Geometry check sheet. Reference: the model listing, model coordinates, mm. Face numbers are marked on the shaded views. A direction names the side the tool comes from. Give positions to 0.01 mm unless a question says otherwise; leave off trailing zeros. Order: outer loops, then holes, each group sorted by start corner. A loop starts at its lowest first (then second) coordinate and runs counter-clockwise, first axis right, second up. Notation, with made-up numbers: M 86.25,-19 L 144.25,-19 A36 cw 144.25,15 Z; hole C 33,-36 d5. An arc over 180 degrees is marked long. Answer as CSV lines item,"result". Start each with the question number.
Q1. Thickness scan on line 1 (Y direction, x = 0, z = 21.25); line 2 (X direction, y = -16, z = -5); line 3 (Z direction, x = 13, y = -18.5). Record the ranges inside material, lowest first.
Q2. Section check B-B, the plane y = -33. Record the boundary of the cut face in (x, z).
Q3. Section check C-C, the plane z = 8. Record the boundary of the cut face in (x, y).
Q4. Section check D-D, the plane x = 0. Record the boundary of the cut face in (y, z) (3 decimals), then the cut area to 3 significant figures.
Q5. Section check A-A, the plane x = 10.5. Record the boundary of the cut face in (y, z), then the cut area to 3 significant figures.
Q6. Go/stop test with flat-tipped pins: pin 1 (2.5 mm diameter, centred on x = 0, y = -30, fed in from -Z); pin 2 (5 mm diameter, centred on y = -23, z = -8.5, fed in from +X); pin 3 (12 mm diameter, centred on x = -2.5, y = -9, fed in from -Z). Record where each tip stops, or that it passes through.
Q7. Set-up check for the marked faces 1 and 2: record each of +Z, -Z, +X, -X, +Y, -Y from which the full face is reachable in a straight line by a thin tool's end or side.
Q8. Mould release check, pull along Z, two halves, no side actions. Record for the marked faces 3, 4, 5 and 6: +Z half, -Z half, draft (parallel to the pull), parting line (faces both ways), or undercut.
```python
from build123d import *

# Parameters (mm, degrees)
SKETCH2_R               = 12.575
BOSS_EXTRUDE1_DEPTH     = 36
SKETCH3_R               = 17.5
CUT_EXTRUDE1_DEPTH      = 26
CUT_EXTRUDE2_REACH      = 68.591
CUT_EXTRUDE2_END_RADIUS = 17.5
SKETCH4_R               = 1.5
CUT_EXTRUDE5_REACH      = 71.976
CUT_EXTRUDE5_END_RADIUS = 17.5
SKETCH7_R               = 1.5
CUT_EXTRUDE6_REACH      = 68.357
CUT_EXTRUDE6_END_RADIUS = 17.5
SKETCH8_R               = 1.5


with BuildPart() as part:
    # Sketch2 → Boss-Extrude1 (new body)
    with BuildSketch(Plane(origin=(0, 0, 0), x_dir=(1, 0, 0), z_dir=(0, 1, 0))):
        Polygon((-23, 7.4), (-15, -23.6), (5, -23.6), (28, -1.26), (18, 15.94), (-13, 24.6), align=None)
        with Locations(Location((0, 0, 0), (0, 0, 270))):
            Circle(SKETCH2_R, mode=Mode.SUBTRACT)
    extrude(amount=-BOSS_EXTRUDE1_DEPTH)

    # Sketch3 → Cut-Extrude1 (cut)
    with BuildSketch(Plane.XZ.offset(36)):
        with Locations(Location((0, 0, 0), (0, 0, 270))):
            Circle(SKETCH3_R)
    extrude(amount=-CUT_EXTRUDE1_DEPTH, mode=Mode.SUBTRACT)

    # Cut-Extrude2: up to this cylinder (the profile starts outside it)
    cut_extrude2_end = Plane(origin=(0, -22.5, 0), z_dir=(0, -1, 0)) * Cylinder(CUT_EXTRUDE2_END_RADIUS, 188.182, mode=Mode.PRIVATE)
    # Sketch4 → Cut-Extrude2 (cut, up to the surface)
    with BuildSketch(Plane(origin=(20.378940986, 0, -11.848221504), x_dir=(-0.5026204573745311, 0, -0.8645071866841925), z_dir=(0.8645071866841925, 0, -0.5026204573745311)), mode=Mode.PRIVATE) as cut_extrude2_sk1:
        with Locations((-0.266923677, -15)):
            Circle(SKETCH4_R)
    cut_extrude2_tool1 = extrude(cut_extrude2_sk1.sketch, amount=-CUT_EXTRUDE2_REACH, mode=Mode.PRIVATE) - cut_extrude2_end
    add(cut_extrude2_tool1.solids().sort_by_distance((20.513102, -15, -11.617464))[0], mode=Mode.SUBTRACT)
    # Sketch4 → Cut-Extrude2 (cut, up to the surface)
    with BuildSketch(Plane(origin=(20.378940986, 0, -11.848221504), x_dir=(-0.5026204573745311, 0, -0.8645071866841925), z_dir=(0.8645071866841925, 0, -0.5026204573745311)), mode=Mode.PRIVATE) as cut_extrude2_sk2:
        with Locations((-0.266923677, -30)):
            Circle(SKETCH4_R)
    cut_extrude2_tool2 = extrude(cut_extrude2_sk2.sketch, amount=-CUT_EXTRUDE2_REACH, mode=Mode.PRIVATE) - cut_extrude2_end
    add(cut_extrude2_tool2.solids().sort_by_distance((20.513102, -30, -11.617464))[0], mode=Mode.SUBTRACT)

    # Cut-Extrude5: up to this cylinder (the profile starts outside it)
    cut_extrude5_end = Plane(origin=(0, -22.5, 0), z_dir=(0, -1, 0)) * Cylinder(CUT_EXTRUDE5_END_RADIUS, 194.952, mode=Mode.PRIVATE)
    # Sketch7 → Cut-Extrude5 (cut, up to the surface)
    with BuildSketch(Plane(origin=(-20.405012126, 0, -11.863379143), x_dir=(-0.5026204573745304, 0, 0.8645071866841929), z_dir=(-0.8645071866841929, 0, -0.5026204573745304)), mode=Mode.PRIVATE) as cut_extrude5_sk1:
        with Locations((0.162917338, -30)):
            Circle(SKETCH7_R)
    cut_extrude5_tool1 = extrude(cut_extrude5_sk1.sketch, amount=-CUT_EXTRUDE5_REACH, mode=Mode.PRIVATE) - cut_extrude5_end
    add(cut_extrude5_tool1.solids().sort_by_distance((-20.486898, -30, -11.722536))[0], mode=Mode.SUBTRACT)
    # Sketch7 → Cut-Extrude5 (cut, up to the surface)
    with BuildSketch(Plane(origin=(-20.405012126, 0, -11.863379143), x_dir=(-0.5026204573745304, 0, 0.8645071866841929), z_dir=(-0.8645071866841929, 0, -0.5026204573745304)), mode=Mode.PRIVATE) as cut_extrude5_sk2:
        with Locations((0.162917338, -15)):
            Circle(SKETCH7_R)
    cut_extrude5_tool2 = extrude(cut_extrude5_sk2.sketch, amount=-CUT_EXTRUDE5_REACH, mode=Mode.PRIVATE) - cut_extrude5_end
    add(cut_extrude5_tool2.solids().sort_by_distance((-20.486898, -15, -11.722536))[0], mode=Mode.SUBTRACT)

    # Cut-Extrude6: up to this cylinder (the profile starts outside it)
    cut_extrude6_end = Plane(origin=(0, -22.5, 0), z_dir=(0, -1, 0)) * Cylinder(CUT_EXTRUDE6_END_RADIUS, 187.714, mode=Mode.PRIVATE)
    # Sketch8 → Cut-Extrude6 (cut, up to the surface)
    with BuildSketch(Plane.XY.offset(23.6), mode=Mode.PRIVATE) as cut_extrude6_sk1:
        with Locations((0, -30)):
            Circle(SKETCH8_R)
    cut_extrude6_tool1 = extrude(cut_extrude6_sk1.sketch, amount=-CUT_EXTRUDE6_REACH, mode=Mode.PRIVATE) - cut_extrude6_end
    add(cut_extrude6_tool1.solids().sort_by_distance((0, -30, 23.6))[0], mode=Mode.SUBTRACT)
    # Sketch8 → Cut-Extrude6 (cut, up to the surface)
    with BuildSketch(Plane.XY.offset(23.6), mode=Mode.PRIVATE) as cut_extrude6_sk2:
        with Locations((0, -15)):
            Circle(SKETCH8_R)
    cut_extrude6_tool2 = extrude(cut_extrude6_sk2.sketch, amount=-CUT_EXTRUDE6_REACH, mode=Mode.PRIVATE) - cut_extrude6_end
    add(cut_extrude6_tool2.solids().sort_by_distance((0, -15, 23.6))[0], mode=Mode.SUBTRACT)


solid = part.part
```
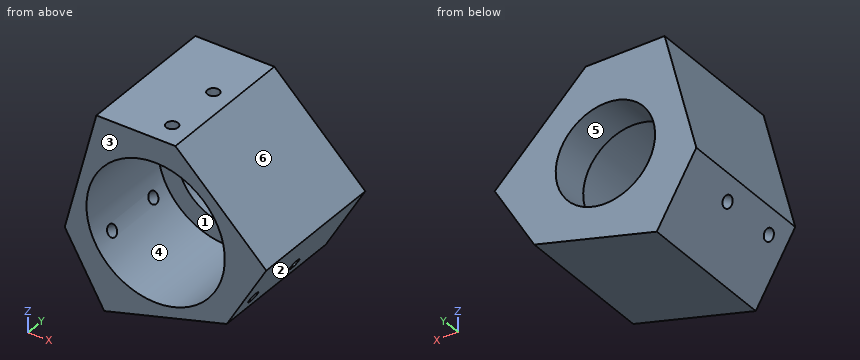
Answer block:
1,line 1,"y = -36 to -31.5, -28.5 to -16.5, -13.5 to 0"
1,line 2,"x = -22.38 to -16.77, 16.77 to 24.36"
1,line 3,"z = -17.34 to -11.72, 11.72 to 15.83"
2,outline,"M -23,-7.4 L -13,-24.6 L 18,-15.94 L 28,1.26 L 5,23.6 L -15,23.6 Z; hole C 0,0 d35"
3,outline,"M -19.03,-36 L -15.56,-36 L -15.56,-10 L -9.7,-10 L -9.7,0 L -19.03,0 Z; M 9.7,-10 L 15.56,-10 L 15.56,-36 L 21.06,-36 L 21.06,0 L 9.7,0 Z"
4,outline,"M -36,-20.968 L 0,-20.968 L 0,-12.575 L -10,-12.575 L -10,-17.5 L -36,-17.5 Z; M -36,17.5 L -31.5,17.5 L -31.5,23.6 L -36,23.6 Z; M -28.5,17.5 L -16.5,17.5 L -16.5,23.6 L -28.5,23.6 Z; M -13.5,17.5 L -10,17.5 L -10,12.575 L 0,12.575 L 0,23.6 L -13.5,23.6 Z"
4,area,"406 mm2"
5,outline,"M -36,-18.04 L 0,-18.04 L 0,-6.92 L -10,-6.92 L -10,-14 L -36,-14 Z; M -36,14 L -10,14 L -10,6.92 L 0,6.92 L 0,18.26 L -36,18.26 Z"
5,area,"440 mm2"
6,pin 1,"stops at z = -21.32"
6,pin 2,"stops at x = 23.78"
6,pin 3,"stops at z = -23.34"
7,face 1,"-Y"
7,face 2,"-Z, +X, +Y, -Y"
8,face 3,"draft"
8,face 4,"undercut"
8,face 5,"undercut"
8,face 6,"+Z half"
